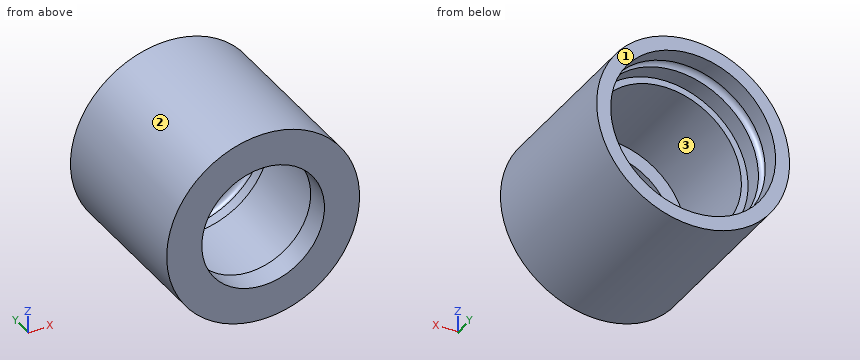
```python
from build123d import *


with BuildPart() as part:
    # Sketch1 → Revolve1 (revolve)
    with BuildSketch(Plane(origin=(0, 0, 0), x_dir=(0, 0, -1), z_dir=(1, 0, 0))):
        with BuildLine():
            Line((0, 0), (0, -88.9))
            Line((0, -88.9), (10.16, -88.9))
            Line((10.16, -88.9), (18.4785, -88.9))
            Line((18.4785, -88.9), (18.4785, -76.2))
            Line((18.4785, -76.2), (10.8585, -76.2))
            Line((10.8585, -76.2), (10.8585, -25.403841866))
            Line((10.8585, -25.403841866), (7.366, -25.403841866))
            Line((7.366, -25.403841866), (7.366, -15.857408119))
            ThreePointArc((7.366, -15.857408119), (4.5593, -12.703841866), (7.366, -9.550275614))
            Line((7.366, -9.550275614), (7.366, 0))
            Line((7.366, 0), (0, 0))
        make_face()
    revolve(axis=Axis((0, -28.313229254, -50.8), (0, -1, 0)))


solid = part.part
```
Model file for the job. Use its own axes, mm. Face numbers are marked on the shaded views. Give positions to 0.01 mm unless a question says otherwise; leave off trailing zeros. Order: outer loops, then holes, each group sorted by start corner. A loop starts at its lowest first (then second) coordinate and runs counter-clockwise, first axis right, second up.
1) Mould opens along Z. For the marked faces 1, 2 and 3 say: +Z half, -Z half, draft (parallel to the pull), parting line (faces both ways), or undercut.
2) Saw through at D-D, the plane y = -42.5. Write the cut outline in (x, z).
3) Wall check: probe 1 along Z at (x, y) = (0, -18.5); probe 2 along X at (y, z) = (-80.25, -50.8); probe 3 along X at (y, z) = (-60.5, -50.8). Give the ranges that are in metal, low to high.
4) Pin check, flat tips, straight feed: pin 1 (1.5 mm diameter, centred on x = -37.5, y = -77, fed in from +Z); pin 2 (6 mm diameter, centred on y = -32.5, z = -67.5, fed in from +X); pin 3 (6 mm diameter, centred on x = -7.5, y = -66, fed in from +Z). Stop position of each tip, or through.
5) Saw through at C-C, the plane y = -21. Write the cut outline in (x, z), then the cut area to 3 significant figures.
Computed:
1. face 1: draft
1. face 2: parting line
1. face 3: undercut
2. outline: circle Ø101.6 at (0, -50.8); hole circle Ø79.88 at (0, -50.8)
3. probe 1: z = -101.6 to -94.23, -7.37 to 0
3. probe 2: x = -50.8 to -32.32, 32.32 to 50.8
3. probe 3: x = -50.8 to -39.94, 39.94 to 50.8
4. pin 1: stops at z = -15.73
4. pin 2: stops at x = 48.92
4. pin 3: stops at z = -0.2
5. outline: circle Ø101.6 at (0, -50.8); hole circle Ø86.87 at (0, -50.8)
5. area: 2,180 mm2
